The listing builds one solid part. Answer for the finished solid, in the listing's coordinates (mm). A direction names the side the tool comes from. Coordinates: 2 decimals unless noted, no trailing zeros. Write each loop counter-clockwise with the first axis right and the second up, starting at its lowest first coordinate (ties: lowest second). Pieces come first, ordered by that corner, then holes.
```python
from build123d import *

# Parameters (mm, degrees)
ESQUISSE1_R        = 4
ESQUISSE1_R_2      = 1
BOSS_EXTRU_1_DEPTH = 5


with BuildPart() as part:
    # Esquisse1 → Boss.-Extru.1 (new body)
    with BuildSketch(Plane(origin=(0, 0, 0), x_dir=(1, 0, 0), z_dir=(0, 1, 0))):
        with BuildLine():
            Line((-32.45676656, 19.27541283), (-5, 12))
            Line((-5, 12), (0, 12))
            ThreePointArc((0, 12), (11.519722281, 3.360952031), (6.452872334, -10.117333574))
            Line((6.452872334, -10.117333574), (-3.66446124, -16.570205908))
            ThreePointArc((-3.66446124, -16.570205908), (-13.815132068, -21.511376537), (-24.82365287, -24.014126066))
            ThreePointArc((-24.82365287, -24.014126066), (-52.345095334, -29.457799684), (-49.895398662, -57.405292665))
            ThreePointArc((-49.895398662, -57.405292665), (-58.555043799, -54.803988162), (-65.722985518, -49.292468357))
            ThreePointArc((-65.722985518, -49.292468357), (-83.868971565, -12.107677443), (-79.535269898, 29.040888933))
            ThreePointArc((-79.535269898, 29.040888933), (-74.684658752, 36.671603877), (-67.436952657, 42.077803594))
            ThreePointArc((-67.436952657, 42.077803594), (-60.180308988, 14.977905063), (-32.45676656, 19.27541283))
        make_face()
        with Locations(Location((0, 0, 0), (0, 0, 270))):
            Circle(ESQUISSE1_R, mode=Mode.SUBTRACT)
        with Locations(Location((7.25, -3.65, 0), (0, 0, 270))):
            Circle(ESQUISSE1_R_2, mode=Mode.SUBTRACT)
        with Locations(Location((7.25, 0, 0), (0, 0, 270))):
            Circle(ESQUISSE1_R_2, mode=Mode.SUBTRACT)
        with Locations(Location((7.25, 3.65, 0), (0, 0, 270))):
            Circle(ESQUISSE1_R_2, mode=Mode.SUBTRACT)
        with Locations(Location((3.65, -7.25, 0), (0, 0, 270))):
            Circle(ESQUISSE1_R_2, mode=Mode.SUBTRACT)
        with Locations(Location((0, -7.25, 0), (0, 0, 270))):
            Circle(ESQUISSE1_R_2, mode=Mode.SUBTRACT)
        with Locations(Location((-3.65, -7.25, 0), (0, 0, 270))):
            Circle(ESQUISSE1_R_2, mode=Mode.SUBTRACT)
        with Locations(Location((-7.25, -3.65, 0), (0, 0, 270))):
            Circle(ESQUISSE1_R_2, mode=Mode.SUBTRACT)
        with Locations(Location((-7.25, 0, 0), (0, 0, 270))):
            Circle(ESQUISSE1_R_2, mode=Mode.SUBTRACT)
        with Locations(Location((-7.25, 3.65, 0), (0, 0, 270))):
            Circle(ESQUISSE1_R_2, mode=Mode.SUBTRACT)
        with Locations(Location((-3.65, 7.25, 0), (0, 0, 270))):
            Circle(ESQUISSE1_R_2, mode=Mode.SUBTRACT)
        with Locations(Location((0, 7.25, 0), (0, 0, 270))):
            Circle(ESQUISSE1_R_2, mode=Mode.SUBTRACT)
        with Locations(Location((3.65, 7.25, 0), (0, 0, 270))):
            Circle(ESQUISSE1_R_2, mode=Mode.SUBTRACT)
    extrude(amount=BOSS_EXTRU_1_DEPTH)


solid = part.part
```
(1) Section A-A, the plane y = 4.15 is taken. State how many separate pieces and enclosed holes the cut face has, plus the area to 3 significant figures.
(2) Each of these flat-tipped pins is pushed along its axis until it touches: pin 1 (2.5 mm diameter, centred on x = 3.65, z = -7.25, fed in from +Y); pin 2 (1.2 mm diameter, centred on x = 3.65, z = 7.25, fed in from +Y); pin 3 (2 mm diameter, centred on x = -20.5, y = 4, fed in from +Z); pin 4 (3 mm diameter, centred on y = 2.5, z = 17.5, fed in from +X). Where does it stop, or does it pass through?
(3) Which of the six approach directions +Z, -Z, +X, -X, +Y, -Y give full straight-line access (tool end or side, diameter ignored) to faces 4 (the flat face through (-3, 2, -12)), 5 (the cylindrical face through (-60.54, 2.46, -15.22))?
(4) Section B-B, the plane z = 12 is taken. Write down the section's boundary in (x, y).
(5) Section C-C, the plane x = -75.5 is taken. Write down the section's boundary in (y, z).
(6) For a pull along X with two mould halves and no side action, classify faces 1 (the flat face through (-47, 5, 7)), 2 (the cylindrical face through (-3.905, 2.465, -0.867)), 3 (the cylindrical face through (-58.442, 2.465, 54.862)) as pulls with the +X half, pulls with the -X half, needs draft (parallel to the pull), parting line crosses it, or undercut.
(7) Find the intervals of material crossed by probe 1 along X at (y, z) = (3.5, 7.25); probe 2 along X at (y, z) = (1.75, -7.25); probe 3 along Z at (x, y) = (0.5, 3.7), in increasing order.
Solution:
1. separate pieces: 1
1. enclosed holes: 13
1. area: 4,100 mm2
2. pin 1: stops at y = 5
2. pin 2: passes through
2. pin 3: stops at z = 23.54
2. pin 4: stops at x = -2.77
3. face 4: -Z, +X, +Y, -Y
3. face 5: +Y, -Y
4. outline: (-83.89, 0) - (3.5, 0) - (3.5, 5) - (-83.89, 5) - close
5. outline: (0, -35.75) - (5, -35.75) - (5, 35.63) - (0, 35.63) - close
6. face 1: needs draft
6. face 2: undercut
6. face 3: pulls with the -X half
7. probe 1: x = -84.56 to -4.65, -2.65 to -1, 1 to 2.65, 4.65 to 9.56
7. probe 2: x = -84.74 to -4.65, -2.65 to -1, 1 to 2.65, 4.65 to 9.56
7. probe 3: z = -11.99 to -8.12, -6.38 to -3.97, 3.97 to 6.38, 8.12 to 13.91
